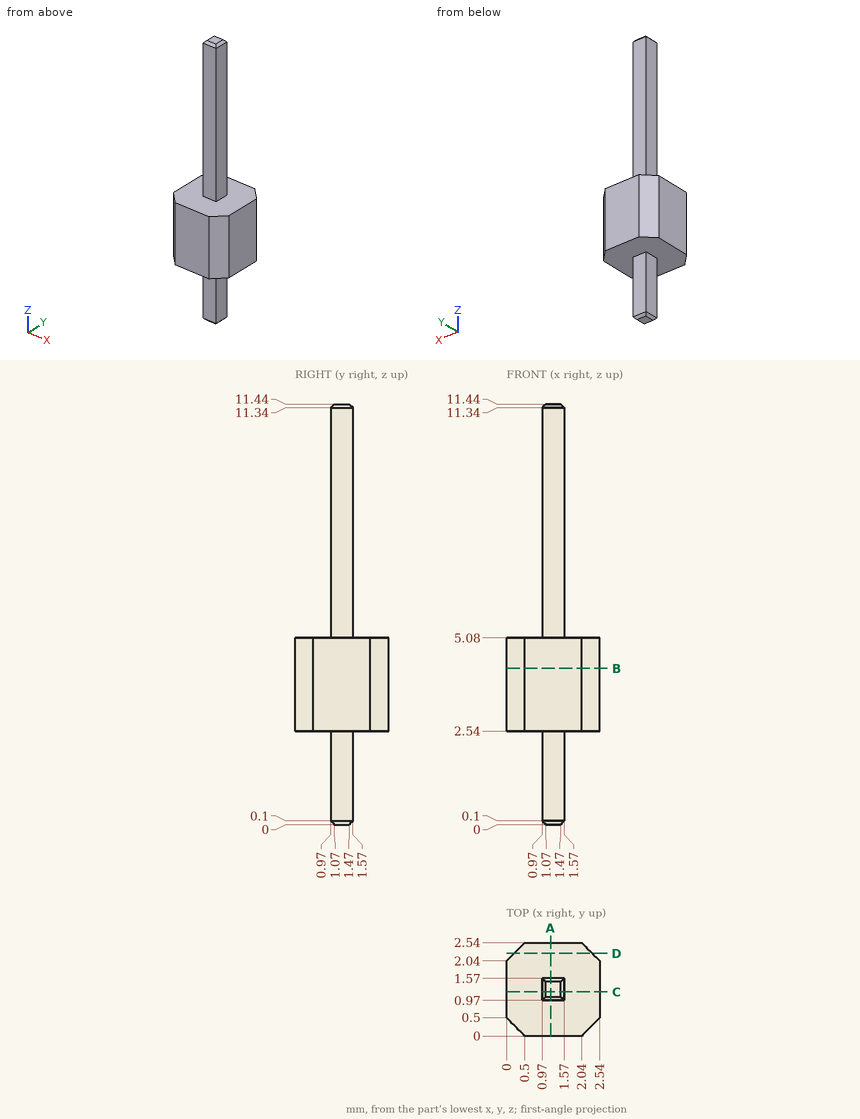
Geometry check sheet. Reference: drawing and pictorial views, mm from the part's lowest x, y, z. Give positions to 0.01 mm unless a question says otherwise; leave off trailing zeros. Loops run counter-clockwise (first coordinate to the right, second up) from the corner with the lowest first, then second, coordinate; pieces in that order, holes last.
1. Go/stop test with flat-tipped pins: pin 1 Ø0.7 at (x, z) = (1, 7.5) entering from -Y; pin 2 Ø0.5 at (y, z) = (1, 9.5) entering from -X; pin 3 Ø0.5 at (y, z) = (1.5, 7) entering from +X; pin 4 Ø1.3 at (x, y) = (1.5, 1) entering from -Z. Record where each tip stops, or that it passes through.
2. Section check A-A, the plane x = 1.2. Enter the section's corners in (y, z).
3. Section check D-D, the plane y = 2.25. Enter the section's corners in (x, z).
4. Thickness scan on line 1 (Z direction, x = 2.2, y = 1.2); line 2 (X direction, y = 1.45, z = 6.25). Record the ranges inside material, lowest first.
5. Section check B-B, the plane z = 4.25. Enter the section's corners in (x, y), then the cut area to 3 significant figures.
Geometry says:
1. pin 1: stops at y = 0.97
1. pin 2: stops at x = 0.97
1. pin 3: stops at x = 1.57
1. pin 4: stops at z = 0
2. outline: (0, 2.54) - (0.97, 2.54) - (0.97, 0.1) - (1.07, 0) - (1.47, 0) - (1.57, 0.1) - (1.57, 2.54) - (2.54, 2.54) - (2.54, 5.08) - (1.57, 5.08) - (1.57, 11.34) - (1.47, 11.44) - (1.07, 11.44) - (0.97, 11.34) - (0.97, 5.08) - (0, 5.08) - close
3. outline: (0.21, 2.54) - (2.33, 2.54) - (2.33, 5.08) - (0.21, 5.08) - close
4. line 1: z = 2.54 to 5.08
4. line 2: x = 0.97 to 1.57
5. outline: (0, 0.5) - (0.5, 0) - (2.04, 0) - (2.54, 0.5) - (2.54, 2.04) - (2.04, 2.54) - (0.5, 2.54) - (0, 2.04) - close
5. area: 5.95 mm2
